Autodesk Inventor part; units mm, degrees
ref_plane "YZ Plane" through (0, 0, 0) normal (1, 0, 0) x (0, 1, 0)
ref_plane "XZ Plane" through (0, 0, 0) normal (0, 1, 0) x (-1, 0, 0)
ref_plane "XY Plane" through (0, 0, 0) normal (0, 0, 1) x (1, 0, 0)
sketch "Boceto1" plane through (0, 0, 0) normal (0, 1, 0) x (-1, 0, 0)
  arc A0 (0, -33) -> (0, 33) centre (0, 0) ccw
  arc A1 (0, -36) -> (0, 36) centre (0, 0) ccw
  arc A2 (0, -42) -> (0, 42) centre (0, 0) ccw
  line L0 (0, -42) -> (0, 42)
  circle A3 centre (177, 0) radius 22
  circle A4 centre (177, 0) radius 18
  line L1 (159.2518, -13) -> (39.9375, -13)
  line L2 (159.2518, 13) -> (39.9375, 13)
  line L3 (139, 0) -> (57, 0) construction
  line L4 (139, 8) -> (57, 8)
  line L5 (57, -8) -> (139, -8)
  arc A5 (139, -8) -> (139, 8) centre (139, 0) ccw
  arc A6 (57, 8) -> (57, -8) centre (57, 0) ccw
  point P0 (98, 0)
  dimension "d0" = 66
  dimension "d1" = 72
  dimension "d2" = 84
  dimension "d3" = 44
  dimension "d4" = 177
  dimension "d5" = 36
  dimension "d6" = 26
  dimension "d7" = 41
  dimension "d8" = 16
  dimension "d9" = 57
extrude "Extrusión1" add sketch "Boceto1" along normal mid plane 38 contours A1 L0 A2
extrude "Extrusión2" add sketch "Boceto1" along normal mid plane 34 contours A0 L0 A1
sketch "Boceto2" plane through (0, -19, -42) normal (1, 0, 0) x (0, 0, -1)
  line L0 (0, 0) -> (0, 38)
  circle A0 centre (0, 19) radius 9
  circle A1 centre (0, 19) radius 6
  point P0 (-42, 19)
  point P1 (0, 25)
  point P2 (0, 13)
  dimension "d18" = 18
  dimension "d19" = 12
extrude "Extrusión5" cut sketch "Boceto2" against normal up to surface contours A1 L0 picked at (-1.87, 18.2908)
extrude "Extrusión6" add sketch "Boceto2" against normal blind 33 contours A0 L0 A1 | L0 A1 A0
mirror "Simetría1" about plane through (0, 0, 0) normal (0, 0, 1) of "Extrusión6", "Extrusión5"
chamfer "Chaflán2" distance 0.5 angle 45 2 edges at (-42, 19, 0) (-42, -19, 0)
properties part number "EM-004" material "Acero, alta resistencia, aleación baja"
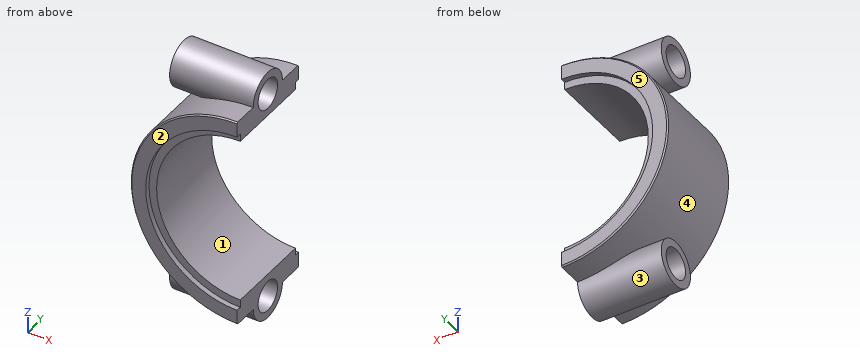
Read the model definition and answer for the solid it produces. Units are mm, in the model's axes. Face numbers are marked on the shaded views. A direction names the side the tool comes from. Round coordinates to 2 decimals unless told otherwise and drop trailing zeros. Write each loop counter-clockwise with the first axis right and the second up, starting at its lowest first coordinate (ties: lowest second). Pieces come first, ordered by that corner, then holes. Notation, with made-up numbers: (57.25, -28.5) - (80.25, -28.5) arc R18 ccw to (80.25, -4.5) - close; hole circle Ø4 at (63.5, 3.5). An arc over 180 degrees is marked (long way). Use a Markdown table: item, result.
(1) The part is cut by section D-D (y = 11). Write down the section's boundary in (x, z), then the cut area to 3 significant figures.
Reported:
| item | result |
|---|---|
| outline | (0, -42) - (0, -33) arc R33 cw to (0, 33) - (0, 42) arc R42 ccw to start |
| area | 1,060 mm2 |
(2) The mould has two halves that part along Z. Classify the marked faces 1, 2 and 3: released by +Z, released by -Z, zero draft, split by the parting line, or undercut.
Reported:
| item | result |
|---|---|
| face 1 | undercut |
| face 2 | zero draft |
| face 3 | undercut |
(3) The part is cut by section A-A (z = 0). Write down the section's boundary in (x, y).
Reported:
| item | result |
|---|---|
| outline | (-42, -18.5) - (-41.5, -19) - (-36, -19) - (-36, -17) - (-33, -17) - (-33, 17) - (-36, 17) - (-36, 19) - (-41.5, 19) - (-42, 18.5) - close |
(4) Which of the six approach directions +Z, -Z, +X, -X, +Y, -Y give full straight-line access (tool end or side, diameter ignored) to the marked faces 4 and 5?
Reported:
| item | result |
|---|---|
| face 4 | -X |
| face 5 | +Z, -Z, +X, -X, +Y |
(5) The part is cut by section C-C (y = -7). Write down the section's boundary in (x, z).
Reported:
| item | result |
|---|---|
| outline | (-33, -47.66) - (0, -47.66) - (0, -33) arc R33 cw to (0, 33) - (0, 47.66) - (-33, 47.66) - (-33, 36.34) - (-21.05, 36.34) arc R42 ccw to (-21.05, -36.34) - (-33, -36.34) - close |
(6) Straight lines are drawn through the part: line 1 along Y through (x, z) = (-14, 42); line 2 along X through (y, z) = (16, 1); line 3 along Z through (x, y) = (-17, 2.5). For each, find the intervals that lie inside material, in ascending order. Write a range as [from, to].
Reported:
| item | result |
|---|---|
| line 1 | [-9, -6], [6, 9] |
| line 2 | [-41.99, -32.98] |
| line 3 | [-50.65, -47.45], [-36.55, -28.28], [28.28, 36.55], [47.45, 50.65] |
(7) Each of these flat-tipped pins is pushed along its axis until it touches: pin 1 Ø14.5 at (y, z) = (0, 43) entering from -X; pin 2 Ø4 at (y, z) = (6.5, 23.5) entering from +X; pin 3 Ø11 at (x, z) = (-26.5, -8.5) entering from -Y; pin 4 Ø12 at (x, z) = (-37, 24.5) entering from -Y. Where does it stop, or does it pass through?
Reported:
| item | result |
|---|---|
| pin 1 | x = -33 |
| pin 2 | x = -20.95 |
| pin 3 | y = -17 |
| pin 4 | y = -19 |
(8) The part is cut by section B-B (y = 0). Write down the section's boundary in (x, z).
Reported:
| item | result |
|---|---|
| outline | (-33, -51) - (0, -51) - (0, -48) - (-33, -48) - close; (-33, -36) - (0, -36) - (0, -33) arc R33 cw to (0, 33) - (0, 36) - (-33, 36) - (-33, 33) - (-25.98, 33) arc R42 ccw to (-25.98, -33) - (-33, -33) - close; (-33, 48) - (0, 48) - (0, 51) - (-33, 51) - close |
